```python
from build123d import *

# Parameters (mm, degrees)
SKETCH1_R                                           = 6.985
BOSS_EXTRUDE1_DEPTH                                 = 11.43
CSK_FOR_1_4_FLAT_HEAD_MACHINE_SCREW_100_D           = 6.35
CSK_FOR_1_4_FLAT_HEAD_MACHINE_SCREW_100_CSINK_D     = 10.16
CSK_FOR_1_4_FLAT_HEAD_MACHINE_SCREW_100_CSINK_ANGLE = 60
CUT_EXTRUDE1_DEPTH                                  = 5.715


with BuildPart() as part:
    # Sketch1 → Boss-Extrude1 (new body)
    with BuildSketch(Plane(origin=(0, 0, 0), x_dir=(1, 0, 0), z_dir=(0, 1, 0))):
        with Locations(Location((0, 0, 0), (0, 0, 270))):
            Circle(SKETCH1_R)
    extrude(amount=BOSS_EXTRUDE1_DEPTH)

    # CSK for 1/4 Flat Head Machine Screw (100)1 (through all)
    with Locations(Plane(origin=(0, 11.43, 0), x_dir=(1, 0, 0), z_dir=(0, 1, 0))):
        with Locations((0, 0)):
            CounterSinkHole(CSK_FOR_1_4_FLAT_HEAD_MACHINE_SCREW_100_D / 2, CSK_FOR_1_4_FLAT_HEAD_MACHINE_SCREW_100_CSINK_D / 2, counter_sink_angle=CSK_FOR_1_4_FLAT_HEAD_MACHINE_SCREW_100_CSINK_ANGLE)

    # Sketch4 → Cut-Extrude1 (cut)
    with BuildSketch(Plane.XZ):
        Polygon((5.43794625, -3.738588047), (5.956685348, 2.840105573), (0.518739098, 6.57869362), (-5.43794625, 3.738588047), (-5.956685348, -2.840105573), (-0.518739098, -6.57869362), align=None)
    extrude(amount=-CUT_EXTRUDE1_DEPTH, mode=Mode.SUBTRACT)


solid = part.part
```
Part model, mm, in its own coordinate system. A direction names the side the tool comes from. Round coordinates to 2 decimals unless told otherwise and drop trailing zeros. Write each loop counter-clockwise with the first axis right and the second up, starting at its lowest first coordinate (ties: lowest second). Pieces come first, ordered by that corner, then holes. Notation, with made-up numbers: M 77.5,-12.5 L 111.5,-12.5 A8 cw 111.5,-1.5 Z; hole C 61,13 d6. An arc over 180 degrees is marked long. Answer as CSV lines item,"result". Start each with the question number.
1) Which spindle directions (+Z, -Z, +X, -X, +Y, -Y) get a long thin tool onto all of the face, cutting with end or side? Do faces 4 (the face through (0.69, 6.91, 3.1)), 5 (the face through (5.694, 2.817, -0.495)). Say none if no direction does.
2) Drill centre lines: L1, parallel to Z at x = -0.75, y = 9.25; L2, parallel to X at y = 5.25, z = 3; L3, parallel to X at y = 6.75, z = 0.25. Where is each one in solid material? Low to high.
3) Mould opens along X. For faces 1 (the face through (6.926, 5.635, -0.909)), 2 (the face through (2.418, 2.817, -5.179)), 3 (the face through (-6, 0, 1)) say: +X half, -X half, draft (parallel to the pull), parting line (faces both ways), or undercut.
4) Band-saw the part on D-D (x = -5.75). List the corners of the cut face in (y, z) (3 decimals).
5) Band-saw the part on A-A (y = 3.25). List the corners of the cut face in (x, z) (3 decimals).
6) Drop flat-ended pins along their axis: pin 1 (1.5 mm diameter, centred on y = 2, z = -5, fed in from -X); pin 2 (1 mm diameter, centred on y = 3.5, z = 4, fed in from -X); pin 3 (1 mm diameter, centred on y = 7, z = -3.5, fed in from +X). Give the stop position or say it passes through.
7) Band-saw the part on C-C (z = 0). List the corners of the cut face in (x, y) (3 decimals), then the cut area to 3 significant figures.
8) Band-saw the part on B-B (x = 0). List the corners of the cut face in (y, z) (3 decimals), then the cut area to 3 significant figures.
Worked out:
1,face 4,"+Y, -Y"
1,face 5,"-Y"
2,L1,"-6.94 to -3.75, 3.75 to 6.94"
2,L2,"-6.31 to -5.5, 5.72 to 6.31"
2,L3,"-6.98 to -3.17, 3.17 to 6.98"
3,face 1,"parting line"
3,face 2,"undercut"
3,face 3,"draft"
4,outline,"M 0,-3.966 L 11.43,-3.966 L 11.43,3.966 L 0,3.966 L 0,-0.219 L 5.715,-0.219 L 5.715,-2.982 L 0,-2.982 Z"
5,outline,"C 0,0 d13.97; hole M -5.957,-2.84 L -0.519,-6.579 L 5.438,-3.739 L 5.957,2.84 L 0.519,6.579 L -5.438,3.739 Z"
6,pin 1,"x = -5.54"
6,pin 2,"x = -6.04"
6,pin 3,"x = 6.31"
7,outline,"M -6.985,0 L -5.733,0 L -5.733,5.715 L -3.175,5.715 L -3.175,8.13 L -5.08,11.43 L -6.985,11.43 Z; M 3.175,5.715 L 5.733,5.715 L 5.733,0 L 6.985,0 L 6.985,11.43 L 5.08,11.43 L 3.175,8.13 Z"
7,area,"51.6 mm²"
8,outline,"M 0,-6.985 L 11.43,-6.985 L 11.43,-5.08 L 8.13,-3.175 L 5.715,-3.175 L 5.715,-6.331 L 0,-6.331 Z; M 0,6.331 L 5.715,6.331 L 5.715,3.175 L 8.13,3.175 L 11.43,5.08 L 11.43,6.985 L 0,6.985 Z"
8,area,"44.7 mm²"
